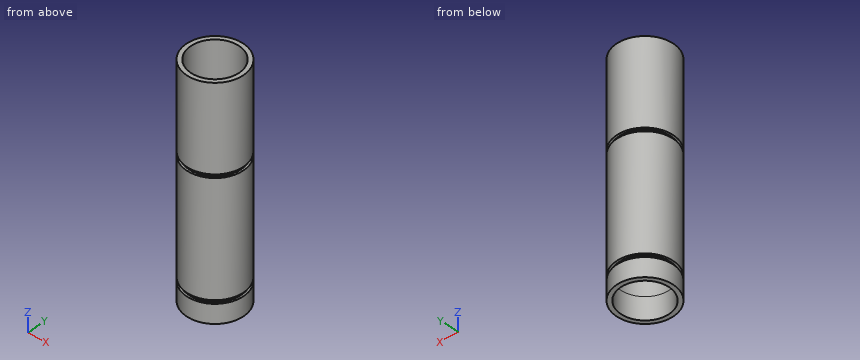
Autodesk Inventor part; units mm, degrees
ref_plane "РабПлоскость2" through (0, 0, 40) normal (0, 0, 1) x (1, 0, 0)
ref_plane "РабПлоскость4" through (0, 0, 0) normal (0, 0, -1) x (-1, 0, 0)
ref_plane "YZ Plane" through (0, 0, 0) normal (1, 0, 0) x (0, 1, 0)
sketch "Эскиз1" plane through (0, 0, 0) normal (0, 0, 1) x (1, 0, 0)
  circle A0 centre (0, 0) radius 10
  circle A1 centre (0, 0) radius 8.5
  dimension "d1" = 20
  dimension "d2" = 17
extrude "Выдавливание1" add sketch "Эскиз1" along normal blind 74
ref_plane "РабПлоскость1" through (0, 0, 33) normal (0, 0, -1) x (-1, 0, 0)
ref_plane "РабПлоскость2" through (0, 0, 40) normal (0, 0, 1) x (1, 0, 0)
sketch "Эскиз3" plane through (0, 0, 40) normal (0, 0, 1) x (1, 0, 0)
  circle A0 centre (0, 0) radius 8.5
  circle A1 centre (0, 0) radius 9.25
  circle A2 centre (0, 0) radius 11
  dimension "d9" = 18.5
  dimension "d10" = 22
extrude "Выдавливание3" cut sketch "Эскиз3" along normal blind 1.2 contours A2
ref_plane "РабПлоскость4" through (0, 0, 0) normal (0, 0, -1) x (-1, 0, 0)
ref_plane "РабПлоскость3" through (0, 0, 7) normal (0, 0, -1) x (-1, 0, 0)
sketch "Эскиз6" plane through (0, 0, 0) normal (0, 0, -1) x (-1, 0, 0)
  circle A0 centre (0, 0) radius 8.5
  circle A1 centre (0, 0) radius 10
extrude "Выдавливание6" add sketch "Эскиз6" along normal blind 15
sketch "Эскиз7" plane through (0, 0, 0) normal (0, 0, -1) x (-1, 0, 0)
  circle A0 centre (0, 0) radius 9.25
  circle A1 centre (0, 0) radius 11
  dimension "d25" = 18.5
  dimension "d26" = 22
extrude "Выдавливание7" cut sketch "Эскиз7" along normal blind 1.2
sketch "Эскиз8" plane through (0, 0, 74) normal (0, 0, 1) x (1, 0, 0)
  circle A0 centre (0, 0) radius 19.934
extrude "Выдавливание8" cut sketch "Эскиз8" against normal blind 2.8
sketch "Эскиз9" plane through (0, 0, -15) normal (0, 0, -1) x (-1, 0, 0)
  circle A0 centre (0, 0) radius 19.6449
  dimension "d33" = 39.2898
extrude "Выдавливание9" cut sketch "Эскиз9" against normal blind 7.2
properties part number "труба"
Here's how the part is built. I have some questions about the finished solid (model axes, mm). Round coordinates to 2 decimals unless told otherwise and drop trailing zeros. Write each loop counter-clockwise with the first axis right and the second up, starting at its lowest first coordinate (ties: lowest second). Pieces come first, ordered by that corner, then holes. Notation, with made-up numbers: M 55.5,44 L 79.5,44 A17 ccw 79.5,72 Z; hole C 36,9 d3. An arc over 180 degrees is marked long. Answer as CSV lines item,"result". Start each with the question number.
1. Suppose I cut it at C-C on z = 45.5. Write out the boundary of the cut face in (x, y).
2. I need wall thicknesses on probe 1 along X at (y, z) = (0, -4); probe 2 along Y at (x, z) = (1.5, 59). Which ranges of each line are inside material? Lowest first, please.
3. I'm going to push flat-ended pins straight in: pin 1 Ø2 at (y, z) = (1.5, 43.5) entering from +X; pin 2 Ø1.5 at (y, z) = (-4, 5.5) entering from -X; pin 3 Ø8 at (y, z) = (5.5, 8) entering from -X. Where does each tip first touch, or does it pass through?
4. Suppose I cut it at B-B on x = -6. Write out the boundary of the cut face in (y, z).
5. Suppose I cut it at A-A on y = 0. Write out the boundary of the cut face in (x, z).
Check result:
1,outline,"C 0,0 d20; hole C 0,0 d17"
2,probe 1,"x = -10 to -8.5, 8.5 to 10"
2,probe 2,"y = -9.89 to -8.37, 8.37 to 9.89"
3,pin 1,"stops at x = 9.99"
3,pin 2,"stops at x = -9.46"
3,pin 3,"stops at x = -9.89"
4,outline,"M -8,-7.8 L -6.02,-7.8 L -6.02,71.2 L -8,71.2 L -8,41.2 L -7.04,41.2 L -7.04,40 L -8,40 L -8,0 L -7.04,0 L -7.04,-1.2 L -8,-1.2 Z; M 6.02,-7.8 L 8,-7.8 L 8,-1.2 L 7.04,-1.2 L 7.04,0 L 8,0 L 8,40 L 7.04,40 L 7.04,41.2 L 8,41.2 L 8,71.2 L 6.02,71.2 Z"
5,outline,"M -10,-7.8 L -8.5,-7.8 L -8.5,71.2 L -10,71.2 L -10,41.2 L -9.25,41.2 L -9.25,40 L -10,40 L -10,0 L -9.25,0 L -9.25,-1.2 L -10,-1.2 Z; M 8.5,-7.8 L 10,-7.8 L 10,-1.2 L 9.25,-1.2 L 9.25,0 L 10,0 L 10,40 L 9.25,40 L 9.25,41.2 L 10,41.2 L 10,71.2 L 8.5,71.2 Z"
